Could you check a few things on this model? Use its own coordinates, in mm. A direction names the side the tool comes from. Round coordinates to 2 decimals unless told otherwise and drop trailing zeros. Write each loop counter-clockwise with the first axis right and the second up, starting at its lowest first coordinate (ties: lowest second). Pieces come first, ordered by that corner, then holes. Notation, with made-up numbers: (-19.5, -31) -> (-6.5, -31) arc R25 cw to (-6.5, 3) -> close; hole circle Ø7 at (20.5, 51). An arc over 180 degrees is marked (long way). Return JSON: item names as keys, results as strings.
Autodesk Inventor part; units mm, degrees
ref_plane "YZ Plane" through (0, 0, 0) normal (1, 0, 0) x (0, 1, 0)
ref_plane "XZ Plane" through (0, 0, 0) normal (0, 1, 0) x (-1, 0, 0)
ref_plane "XY Plane" through (0, 0, 0) normal (0, 0, 1) x (1, 0, 0)
sketch "Sketch1" plane through (0, 0, 0) normal (0, 0, 1) x (1, 0, 0)
  circle A0 centre (0, 0) radius 18.1864 construction
  circle A1 centre (-61.1981, 101.1124) radius 54.5719 construction
  line L0 (-61.1981, 101.1124) -> (0, 0) construction
  arc A2 (-12.3694, 112.6139) -> (-94.0337, 63.1868) centre (-61.1981, 101.1124) ccw
  arc A3 (-9.0194, -10.4175) -> (13.4124, 3.1593) centre (0, 0) ccw
  line L1 (-94.0337, 63.1868) -> (-9.0194, -10.4175)
  line L2 (-12.3694, 112.6139) -> (13.4124, 3.1593)
  line L3 (-14.7885, -17.0809) -> (-99.8028, 56.5234)
  arc A4 (-3.7904, 114.6347) -> (-99.8028, 56.5234) centre (-61.1981, 101.1124) ccw
  line L4 (-3.7904, 114.6347) -> (21.9915, 5.1801)
  arc A5 (-14.7885, -17.0809) -> (21.9915, 5.1801) centre (0, 0) ccw
  line L5 (-11.9039, -13.7492) -> (-96.9182, 59.8551) construction
  arc A6 (-8.0799, 113.6243) -> (-96.9182, 59.8551) centre (-61.1981, 101.1124) ccw construction
  line L6 (-8.0799, 113.6243) -> (17.7019, 4.1697) construction
  arc A7 (-11.9039, -13.7492) -> (17.7019, 4.1697) centre (0, 0) ccw construction
  dimension "d0" = 36.3728
  dimension "d1" = 109.1438
  dimension "d2" = 118.1902
  dimension "d3" = 8.8138
  dimension "d4" = 61.1981
  dimension "d5" = 4.4069
extrude "Extrusion1" add sketch "Sketch1" along normal mid plane 11.8364
equation "\"d5\" = 0.5 * d3"
properties part number "EL2-CGB-009" material "Steel"
1) Will these pins go through, and if not, where does the flat tip stop? pin 1 Ø6 at (x, z) = (-101.5, -4) entering from -Y; pin 2 Ø2 at (x, z) = (-71.5, -2) entering from -Y; pin 3 Ø1 at (x, z) = (-70.5, -0.5) entering from +Y.
Return value:
{"pin 1": "y = 55.4", "pin 2": "y = 31.15", "pin 3": "y = 159.43"}
2) For faces 4 (the face through (-56.701, 19.206, -0.083)), 5 (the face through (-52.12, 26.9, -0.08)), which set-ups out of +Z, -Z, +X, -X, +Y, -Y let a thin tool reach every point of the face, with its end or its side?
Return value:
{"face 4": "+Z, -Z, -X, -Y", "face 5": "+Z, -Z"}
3) I want a section at B-B, the plane z = 2. Please give me the cut outline in (x, y) (1 decimal).
Return value:
{"outline": "(-99.8, 56.5) -> (-14.8, -17.1) arc R22.6 ccw to (22, 5.2) -> (-3.8, 114.6) arc R59 ccw (long way) to start; hole (-94, 63.2) -> (-9, -10.4) arc R13.8 ccw to (13.4, 3.2) -> (-12.4, 112.6) arc R50.2 ccw (long way) to start"}
4) If I drill on probe 1 along X at (y, z) = (45, -2.5); probe 2 along Y at (x, z) = (-100, 1.5); probe 3 along Y at (x, z) = (-87, 3.5), over which ranges is the centre line in solid material (lowest first)? Write a range as [from, to].
Return value:
{"probe 1": "[-86.49, -73.03], [3.56, 12.61]", "probe 2": "[56.69, 69.32], [132.91, 145.53]", "probe 3": "[45.44, 57.1], [144.13, 154.15]"}
5) Thinking about a two-plate mould opening in Y: for faces 1 (the face through (8.92, 60.67, -0.08)), 2 (the face through (0.34, 58.65, -0.08)), 3 (the face through (-70, 42, 5.918)), which applies, pulls with the +Y half, pulls with the -Y half, needs draft (parallel to the pull), parting line crosses it, or undercut?
Return value:
{"face 1": "pulls with the +Y half", "face 2": "undercut", "face 3": "needs draft"}
6) I want a section at A-A, the plane y = 124.5. Please give me the cut outline in (x, z).
Return value:
{"outline": "(-115.34, -5.92) -> (-105.58, -5.92) -> (-105.58, 5.92) -> (-115.34, 5.92) -> close; (-16.82, -5.92) -> (-7.05, -5.92) -> (-7.05, 5.92) -> (-16.82, 5.92) -> close"}
7) I want a section at C-C, the plane x = -108.5. Please give me the cut outline in (y, z).
Return value:
{"outline": "(65.88, -5.92) -> (84.41, -5.92) -> (84.41, 5.92) -> (65.88, 5.92) -> close; (117.82, -5.92) -> (136.34, -5.92) -> (136.34, 5.92) -> (117.82, 5.92) -> close"}
